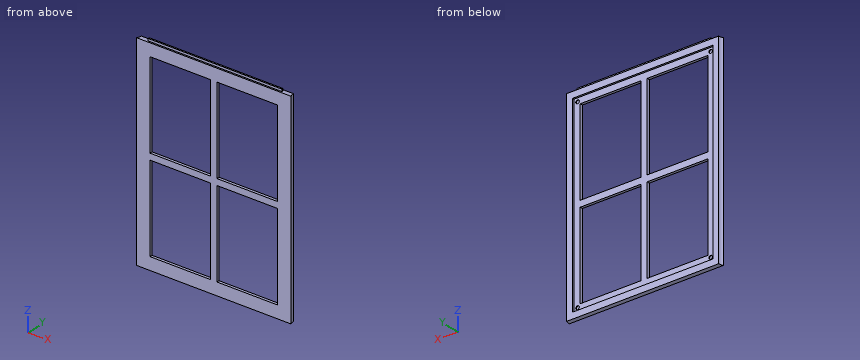
from build123d import *

# Parameters (mm, degrees)
ESBO_O2_W                = 150
ESBO_O2_H                = 2
RESSALTO_EXTRUS_O1_DEPTH = 230
ESBO_O4_W                = 149.6
ESBO_O4_H                = 1.6
RESSALTO_EXTRUS_O2_DEPTH = 2.48
ESBO_O6_W                = 150
ESBO_O6_H                = 2
RESSALTO_EXTRUS_O4_DEPTH = 230
ESBO_O3_W                = 156.68
ESBO_O3_H                = 216
CORTE_EXTRUS_O6_DEPTH    = 2
ESBO_O8_W                = 67.84
ESBO_O8_H                = 97.5
CORTE_EXTRUS_O7_DEPTH    = 20
ESBO_O14_R               = 2
CORTE_EXTRUS_O9_DEPTH    = 1


with BuildPart() as part:
    # Esbo_o2 → Ressalto-extrus_o1 (new body)
    with BuildSketch(Plane.XY):
        with BuildLine():
            Line((-158.025595127, 4.746007498), (11.974404873, 4.746007498))
            ThreePointArc((11.974404873, 4.746007498), (12.315146611, 2.157817047), (13.314150836, -0.253992502))
            Line((13.314150836, -0.253992502), (-159.365341089, -0.253992502))
            ThreePointArc((-159.365341089, -0.253992502), (-158.366336864, 2.157817047), (-158.025595127, 4.746007498))
        make_face()
        with Locations((-73.025595127, 2.246007498)):
            Rectangle(ESBO_O2_W, ESBO_O2_H, mode=Mode.SUBTRACT)
    extrude(amount=RESSALTO_EXTRUS_O1_DEPTH)



with BuildPart() as body_2:
    # Esbo_o4 → Ressalto-extrus_o2 (new body)
    with BuildSketch(Plane.XY.offset(230)):
        with Locations((-73.025595127, 2.246007498)):
            Rectangle(ESBO_O4_W, ESBO_O4_H)
    extrude(amount=RESSALTO_EXTRUS_O2_DEPTH)


with BuildPart() as part_1:
    add(part.part)

    add(body_2.part)  # Ressalto-extrus_o4 merges body 2
    # Esbo_o6 → Ressalto-extrus_o4 (add)
    with BuildSketch(Plane(origin=(0, 0, 0), x_dir=(-1, 0, 0), z_dir=(0, 0, -1))):
        with Locations((73.025595127, 2.246007498)):
            Rectangle(ESBO_O6_W, ESBO_O6_H)
    extrude(amount=-RESSALTO_EXTRUS_O4_DEPTH)

    # Esbo_o3 → Corte-extrus_o6 (cut)
    with BuildSketch(Plane.XZ.offset(-4.746007498)):
        with Locations((-73.025595127, 115)):
            Rectangle(ESBO_O3_W, ESBO_O3_H)
    extrude(amount=CORTE_EXTRUS_O6_DEPTH, mode=Mode.SUBTRACT)

    # Esbo_o8 → Corte-extrus_o7 (cut)
    with BuildSketch(Plane(origin=(0, 2.746007498, 0), x_dir=(1, 0, 0), z_dir=(0, 1, 0))):
        with Locations((-110.445595127, -62.75)):
            Rectangle(ESBO_O8_W, ESBO_O8_H)
        with Locations((-35.605595127, -62.75)):
            Rectangle(ESBO_O8_W, ESBO_O8_H)
        with Locations((-110.445595127, -167.25)):
            Rectangle(ESBO_O8_W, ESBO_O8_H)
        with Locations((-35.605595127, -167.25)):
            Rectangle(ESBO_O8_W, ESBO_O8_H)
    extrude(amount=-CORTE_EXTRUS_O7_DEPTH, mode=Mode.SUBTRACT)

    # Esbo_o14 → Corte-extrus_o9 (cut)
    with BuildSketch(Plane(origin=(0, 2.746007498, 0), x_dir=(1, 0, 0), z_dir=(0, 1, 0))):
        with Locations(Location((-147.365595127, -11, 0), (0, 0, 270))):
            Circle(ESBO_O14_R)
        with Locations(Location((1.314404873, -11, 0), (0, 0, 270))):
            Circle(ESBO_O14_R)
        with Locations(Location((-147.365595127, -219, 0), (0, 0, 270))):
            Circle(ESBO_O14_R)
        with Locations(Location((1.314404873, -219, 0), (0, 0, 270))):
            Circle(ESBO_O14_R)
    extrude(amount=-CORTE_EXTRUS_O9_DEPTH, mode=Mode.SUBTRACT)


solid = part_1.part
Can you work these out from the model? Positions are in its coordinate system, mm. Give positions to 0.01 mm unless a question says otherwise; leave off trailing zeros. Order: outer loops, then holes, each group sorted by start corner. A loop starts at its lowest first (then second) coordinate and runs counter-clockwise, first axis right, second up. Notation, with made-up numbers: M 64.25,24.5 L 107.25,24.5 A21 ccw 107.25,59.5 Z; hole C -15,-2 d5. An arc over 180 degrees is marked long. Use one line per item in the form item = value. Start each with the question number.
Item 1: Will these pins go through, and if not, where does the flat tip stop? pin 1 Ø0.8 at (y, z) = (2.5, 230.5) entering from +X; pin 2 Ø4.5 at (x, z) = (-147.5, 219.5) entering from +Y; pin 3 Ø1.2 at (x, z) = (-101, 231.5) entering from -Y.
Item 2: If we section it at A-A (z = 44.5): Write out the boundary of the cut face in (x, y), then the cut area to 3 significant figures.
Item 3: If we section it at C-C (y = 3.9): Write out the boundary of the cut face in (x, z), then the cut area to 3 significant figures.
Item 4: If we section it at B-B (x = -22.5): Write out the boundary of the cut face in (y, z).
Item 5: If I drill on line 1 along Z through (x, y) = (-86, 0.75); line 2 along Z through (x, y) = (-121, 2.3); line 3 along Z through (x, y) = (-102.5, 4.4), over which ranges is the centre line in solid material (lowest first)?
Outcome:
q1.pin_1 = 1.77
q1.pin_2 = 2.75
q1.pin_3 = 1.45
q2.outline = M -159.37,-0.25 L -144.37,-0.25 L -144.37,2.75 L -151.37,2.75 L -151.37,4.75 L -158.03,4.75 A10 cw Z; M -76.53,-0.25 L -69.53,-0.25 L -69.53,2.75 L -76.53,2.75 Z; M -1.69,-0.25 L 13.31,-0.25 A10 cw 11.97,4.75 L 5.31,4.75 L 5.31,2.75 L -1.69,2.75 Z
q2.area = 134 mm2
q3.outline = M -158.06,0 L 12.01,0 L 12.01,230 L -158.06,230 Z; hole M -151.37,7 L 5.31,7 L 5.31,223 L -151.37,223 Z
q3.area = 5,270 mm2
q4.outline = M -0.25,0 L 4.75,0 L 4.75,7 L 2.75,7 L 2.75,14 L -0.25,14 Z; M -0.25,111.5 L 2.75,111.5 L 2.75,118.5 L -0.25,118.5 Z; M -0.25,216 L 2.75,216 L 2.75,223 L 4.75,223 L 4.75,230 L 3.05,230 L 3.05,232.48 L 1.45,232.48 L 1.45,230 L -0.25,230 Z
q5.line_1 = 0 to 14, 111.5 to 118.5, 216 to 230
q5.line_2 = 0 to 14, 111.5 to 118.5, 216 to 232.48
q5.line_3 = 0 to 7, 223 to 230
